Geometry check sheet. Reference: the model listing, model coordinates, mm. Round coordinates to 2 decimals unless told otherwise and drop trailing zeros.
(1) Thickness scan on L1, parallel to Z at x = -67, y = -1.6; L2, parallel to Z at x = 74, y = -2.9; L3, parallel to X at y = -1.8, z = 23. Record the ranges inside material, lowest first.
(2) Draft check along X on faces 1 (the face through (135.058, -1.565, 0.223)), 2 (the face through (-2, -3.175, 1)). Enter one of: pulls with the +X half, pulls with the -X half, needs draft (parallel to the pull), parting line crosses it, or undercut.
(3) Cross-section at A-A on y = -1.7. Count the separate pieces of the cut face and the enclosed holes in it, and give its area (3 significant figures).
(4) Gauge pin test, flat end, axial feed: P1, Ø2.5, axis at x = 60.32, z = -19.35, coming from the -Y side. Record the tip position at first contact, or that the pin passes through.
from build123d import *

# Parameters (mm, degrees)
F0_W     = 300
F0_H     = 101.6
F0_R     = 1.64084
F0_W_2   = 14.666667
F0_H_2   = 3.175
F0_R_2   = 3.2385
F1_DEPTH = 3.175


with BuildPart() as f1:
    # F0 (on Front) → F1 (new body)
    with BuildSketch(Plane.XZ):
        Rectangle(F0_W, F0_H)
        with Locations((-100.9747, -28.25)):
            Circle(F0_R, mode=Mode.SUBTRACT)
        with Locations((-66.447916, -45.085)):
            Rectangle(F0_W_2, F0_H_2, mode=Mode.SUBTRACT)
        Polygon((-23.395833, -46.6725), (-29.78125, -46.6725), (-38.0625, -46.6725), (-44.447917, -46.6725), (-44.447917, -43.4975), (-38.0625, -43.4975), (-29.78125, -43.4975), (-23.395833, -43.4975), align=None, mode=Mode.SUBTRACT)
        with Locations((-1.395834, -45.085)):
            Rectangle(F0_W_2, F0_H_2, mode=Mode.SUBTRACT)
        with Locations((-74.0253, -28.25)):
            Circle(F0_R, mode=Mode.SUBTRACT)
        with Locations((74.0253, -28.25)):
            Circle(F0_R, mode=Mode.SUBTRACT)
        with Locations((69.203551, -25.686205)):
            Circle(F0_R, mode=Mode.SUBTRACT)
        with Locations((84.245844, -32.071352)):
            Circle(F0_R, mode=Mode.SUBTRACT)
        with Locations((89.566855, -33.299827)):
            Circle(F0_R, mode=Mode.SUBTRACT)
        with Locations((94.974686, -34.059871)):
            Circle(F0_R, mode=Mode.SUBTRACT)
        with Locations((100.428181, -34.345699)):
            Circle(F0_R, mode=Mode.SUBTRACT)
        with Locations((105.885835, -34.155135)):
            Circle(F0_R, mode=Mode.SUBTRACT)
        with Locations((111.306113, -33.489631)):
            Circle(F0_R, mode=Mode.SUBTRACT)
        with Locations((79.05215, -30.383795)):
            Circle(F0_R, mode=Mode.SUBTRACT)
        with Locations((100.9747, -28.25)):
            Circle(F0_R, mode=Mode.SUBTRACT)
        with Locations((116.647762, -32.354251)):
            Circle(F0_R, mode=Mode.SUBTRACT)
        with Locations((121.87013, -30.757637)):
            Circle(F0_R, mode=Mode.SUBTRACT)
        with Locations((64.6236, -22.711924)):
            Circle(F0_R, mode=Mode.SUBTRACT)
        with Locations((60.320302, -19.349791)):
            Circle(F0_R, mode=Mode.SUBTRACT)
        with Locations((56.32641, -15.625395)):
            Circle(F0_R, mode=Mode.SUBTRACT)
        with Locations((52.672317, -11.567081)):
            Circle(F0_R, mode=Mode.SUBTRACT)
        with Locations((49.385835, -7.205735)):
            Circle(F0_R, mode=Mode.SUBTRACT)
        with Locations((-100.9747, 28.25)):
            Circle(F0_R, mode=Mode.SUBTRACT)
        with Locations((-74.0253, 28.25)):
            Circle(F0_R, mode=Mode.SUBTRACT)
        with Locations((-66.447916, 45.085)):
            Rectangle(F0_W_2, F0_H_2, mode=Mode.SUBTRACT)
        Polygon((-23.395833, 46.6725), (-23.395833, 43.4975), (-29.78125, 43.4975), (-38.0625, 43.4975), (-44.447917, 43.4975), (-44.447917, 46.6725), (-38.0625, 46.6725), (-29.78125, 46.6725), align=None, mode=Mode.SUBTRACT)
        with Locations((-1.395834, 45.085)):
            Rectangle(F0_W_2, F0_H_2, mode=Mode.SUBTRACT)
        with Locations((49.385835, 7.205735)):
            Circle(F0_R, mode=Mode.SUBTRACT)
        with Locations((52.672317, 11.567081)):
            Circle(F0_R, mode=Mode.SUBTRACT)
        with Locations((56.32641, 15.625395)):
            Circle(F0_R, mode=Mode.SUBTRACT)
        with Locations((60.320302, 19.349791)):
            Circle(F0_R, mode=Mode.SUBTRACT)
        with Locations((64.6236, 22.711924)):
            Circle(F0_R, mode=Mode.SUBTRACT)
        with Locations((138.292953, 0.08036)):
            Circle(F0_R_2, mode=Mode.SUBTRACT)
        with Locations((69.203551, 25.686205)):
            Circle(F0_R, mode=Mode.SUBTRACT)
        with Locations((74.0253, 28.25)):
            Circle(F0_R, mode=Mode.SUBTRACT)
        with Locations((79.05215, 30.383795)):
            Circle(F0_R, mode=Mode.SUBTRACT)
        with Locations((100.9747, 28.25)):
            Circle(F0_R, mode=Mode.SUBTRACT)
        with Locations((84.245844, 32.071352)):
            Circle(F0_R, mode=Mode.SUBTRACT)
        with Locations((89.566855, 33.299827)):
            Circle(F0_R, mode=Mode.SUBTRACT)
        with Locations((94.974686, 34.059871)):
            Circle(F0_R, mode=Mode.SUBTRACT)
        with Locations((100.428181, 34.345699)):
            Circle(F0_R, mode=Mode.SUBTRACT)
        with Locations((105.885835, 34.155135)):
            Circle(F0_R, mode=Mode.SUBTRACT)
        with Locations((111.306113, 33.489631)):
            Circle(F0_R, mode=Mode.SUBTRACT)
        with Locations((121.87013, 30.757637)):
            Circle(F0_R, mode=Mode.SUBTRACT)
        with Locations((116.647762, 32.354251)):
            Circle(F0_R, mode=Mode.SUBTRACT)
    extrude(amount=F1_DEPTH)


solid = f1.part
Found:
1. L1: z = -50.8 to -46.67, -43.5 to 43.5, 46.67 to 50.8
1. L2: z = -50.8 to -29.89, -26.61 to 26.61, 29.89 to 50.8
1. L3: x = -150 to 63.01, 66.24 to 150
2. face 1: undercut
2. face 2: needs draft
3. separate pieces: 1
3. enclosed holes: 45
3. area: 29,800 mm2
4. P1: passes through
